For this review, use the dimensioned drawing (mm, ordinates from the lowest corner) and the shaded views. Give positions to 0.01 mm unless a question says otherwise; leave off trailing zeros. Order: outer loops, then holes, each group sorted by start corner. A loop starts at its lowest first (then second) coordinate and runs counter-clockwise, first axis right, second up. Notation, with made-up numbers: M -37,63.25 L -31,63.25 A6 cw -31,72.25 Z; hole C 80,44 d8. An arc over 180 degrees is marked long. Use CSV: the item, a comma, the result in double quotes. Start each with the question number.
(1) Clearance check with flat-ended pins moving along their axes: P1, Ø0.8, axis at x = 25, z = 1.5, coming from the -Y side; P2, Ø1.1, axis at x = 7.5, z = 1.5, coming from the -Y side; P3, Ø1.1, axis at x = 24, z = 1.5, coming from the +Y side; P4, Ø1.1, axis at x = 15.5, z = 1.5, coming from the -Y side. State where each tip first meets the part, or that it passes through.
(2) Wall thickness on L1, parallel to Y at x = 16, z = 0.45; L2, parallel to X at y = 17.5, z = 0.85; L3, parallel to X at y = 27, z = 1.65: over which ranges is each line inside the solid? List them lowest first. Write a range as from..to.
(3) Consider section A-A (x = 16). Write out the cut boundary in (y, z), and give its area (3 significant figures).
(4) Consider section C-C (z = 1.7). Write out the cut boundary in (x, y).
(5) Draft analysis for pull direction X (two halves, no side actions). For the marked faces 1, 2 and 3, state which applies: pulls with the +X half, pulls with the -X half, needs draft (parallel to the pull), parting line crosses it, or undercut.
(6) Consider section D-D (x = 29.5). Write out the cut boundary in (y, z), and give its area (3 significant figures).
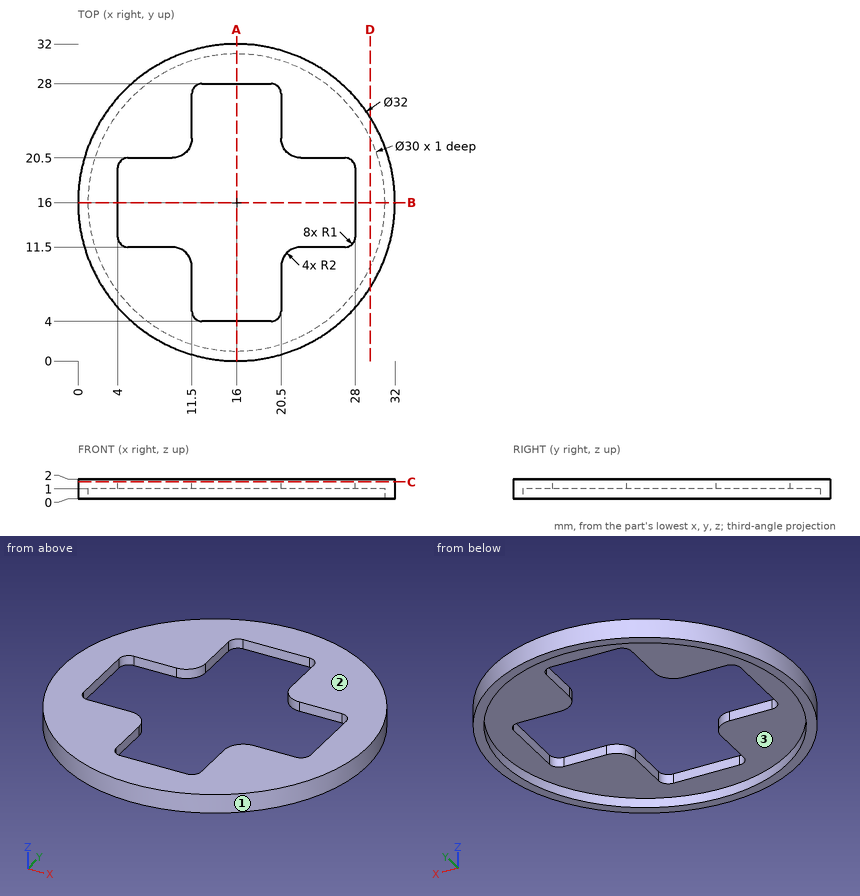
Check result:
1,P1,"stops at y = 2.51"
1,P2,"stops at y = 2.11"
1,P3,"stops at y = 30.16"
1,P4,"stops at y = 0"
2,L1,"y = 0..1, 31..32"
2,L2,"x = 0.07..1.08, 30.92..31.93"
2,L3,"x = 4.38..11.5, 20.5..27.62"
3,outline,"M 0,0 L 1,0 L 1,1 L 4,1 L 4,2 L 0,2 Z; M 28,1 L 31,1 L 31,0 L 32,0 L 32,2 L 28,2 Z"
3,area,"10.0 mm^2"
4,outline,"C 16,16 d32; hole M 4,12.5 A1 ccw 5,11.5 L 9.5,11.5 A2 cw 11.5,9.5 L 11.5,5 A1 ccw 12.5,4 L 19.5,4 A1 ccw 20.5,5 L 20.5,9.5 A2 cw 22.5,11.5 L 27,11.5 A1 ccw 28,12.5 L 28,19.5 A1 ccw 27,20.5 L 22.5,20.5 A2 cw 20.5,22.5 L 20.5,27 A1 ccw 19.5,28 L 12.5,28 A1 ccw 11.5,27 L 11.5,22.5 A2 cw 9.5,20.5 L 5,20.5 A1 ccw 4,19.5 Z"
5,face 1,"parting line crosses it"
5,face 2,"needs draft"
5,face 3,"undercut"
6,outline,"M 7.41,0 L 9.46,0 L 9.46,1 L 22.54,1 L 22.54,0 L 24.59,0 L 24.59,2 L 7.41,2 Z"
6,area,"21.3 mm^2"
